Verification items for the finished model (mm, model axes). A direction names the side the tool comes from. Coordinates: 2 decimals unless noted, no trailing zeros. Order: outer loops, then holes, each group sorted by start corner. A loop starts at its lowest first (then second) coordinate and runs counter-clockwise, first axis right, second up. Notation, with made-up numbers: (76.5, 46) -> (107.5, 46) arc R26 ccw to (107.5, 67) -> close; hole circle Ø3 at (79, -7.75). An arc over 180 degrees is marked (long way). Answer as CSV lines item,"result".
```python
from build123d import *

# Parameters (mm, degrees)
SKETCH_W        = 117
SKETCH_H        = 62
SKETCH_R        = 2
SKETCH_R_2      = 12
PAD_DEPTH       = 2
SKETCH001_W     = 114.9
SKETCH001_H     = 57.8
SKETCH001_W_2   = 110.9
SKETCH001_H_2   = 53.8
SKETCH001_W_3   = 2
SKETCH001_H_3   = 2.1
PAD001_DEPTH    = 2
SKETCH003_R     = 2
POCKET_DEPTH    = 2
SKETCH005_W     = 2
SKETCH005_H     = 62
PAD002_DEPTH    = 19.9
SKETCH006_W     = 2
SKETCH006_H     = 17
POCKET001_DEPTH = 15
SKETCH007_W     = 2
SKETCH007_H     = 15
POCKET002_DEPTH = 17
SKETCH008_R     = 4
SKETCH008_R_2   = 2
PAD003_DEPTH    = 2
SKETCH009_R     = 1.5
POCKET003_DEPTH = 5


with BuildPart() as part:
    # Sketch → Pad (new body)
    with BuildSketch(Plane.XY):
        with Locations((58.5, 31)):
            Rectangle(SKETCH_W, SKETCH_H)
        with Locations((38, 43)):
            Circle(SKETCH_R, mode=Mode.SUBTRACT)
        with Locations((62, 43)):
            Circle(SKETCH_R, mode=Mode.SUBTRACT)
        with Locations((38, 19)):
            Circle(SKETCH_R, mode=Mode.SUBTRACT)
        with Locations((62, 19)):
            Circle(SKETCH_R, mode=Mode.SUBTRACT)
        with Locations((50, 31)):
            Circle(SKETCH_R_2, mode=Mode.SUBTRACT)
        with BuildLine():
            ThreePointArc((71.5, 20), (70, 21.5), (68.5, 20))
            Line((68.5, 20), (68.5, 4))
            ThreePointArc((68.5, 4), (70, 2.5), (71.5, 4))
            Line((71.5, 20), (71.5, 4))
        make_face(mode=Mode.SUBTRACT)
    extrude(amount=PAD_DEPTH)

    # Sketch001 (on Face14 of Pad) → Pad001 (join)
    with BuildSketch(Plane(origin=(0, 0, 0), x_dir=(1, 0, 0), z_dir=(0, 0, -1))):
        with Locations((59.55, -31)):
            Rectangle(SKETCH001_W, SKETCH001_H)
        with Locations((59.55, -31)):
            Rectangle(SKETCH001_W_2, SKETCH001_H_2, mode=Mode.SUBTRACT)
        with Locations((116, -1.05)):
            Rectangle(SKETCH001_W_3, SKETCH001_H_3)
        with Locations((116, -60.95)):
            Rectangle(SKETCH001_W_3, SKETCH001_H_3)
    extrude(amount=PAD001_DEPTH)

    # Sketch003 → Pocket (cut)
    with BuildSketch(Plane.XY.offset(2)):
        with Locations((6, 64)):
            Circle(SKETCH003_R)
        with Locations((113, 64)):
            Circle(SKETCH003_R)
        with Locations((6, -2)):
            Circle(SKETCH003_R)
        with Locations((113, -2)):
            Circle(SKETCH003_R)
    extrude(amount=-POCKET_DEPTH, mode=Mode.SUBTRACT)

    # Sketch005 (on Face16 of Pad001) → Pad002 (join)
    with BuildSketch(Plane(origin=(0, 0, -2), x_dir=(1, 0, 0), z_dir=(0, 0, -1))):
        with Locations((116, -31)):
            Rectangle(SKETCH005_W, SKETCH005_H)
    extrude(amount=PAD002_DEPTH)

    # Sketch006 (on Face37 of Pad002) → Pocket001 (cut)
    with BuildSketch(Plane(origin=(0, 0, -21.9), x_dir=(1, 0, 0), z_dir=(0, 0, -1))):
        with Locations((116, -12.5)):
            Rectangle(SKETCH006_W, SKETCH006_H)
    extrude(amount=-POCKET001_DEPTH, mode=Mode.SUBTRACT)

    # Sketch007 (on Face41 of Pocket001) → Pocket002 (cut)
    with BuildSketch(Plane(origin=(0, 0, -21.9), x_dir=(1, 0, 0), z_dir=(0, 0, -1))):
        with Locations((116, -32)):
            Rectangle(SKETCH007_W, SKETCH007_H)
        with Locations((116, -50)):
            Rectangle(SKETCH007_W, SKETCH007_H)
    extrude(amount=-POCKET002_DEPTH, mode=Mode.SUBTRACT)

    # Sketch008 (on Face4 of Pocket002) → Pad003 (join)
    with BuildSketch(Plane.XY.offset(2)):
        with Locations((6, 64)):
            Circle(SKETCH008_R)
        with Locations((6, 64)):
            Circle(SKETCH008_R_2, mode=Mode.SUBTRACT)
        with Locations((111, 64)):
            Circle(SKETCH008_R)
        with Locations((111, 64)):
            Circle(SKETCH008_R_2, mode=Mode.SUBTRACT)
        with Locations((6, -2)):
            Circle(SKETCH008_R)
        with Locations((6, -2)):
            Circle(SKETCH008_R_2, mode=Mode.SUBTRACT)
        with Locations((111, -2)):
            Circle(SKETCH008_R)
        with Locations((111, -2)):
            Circle(SKETCH008_R_2, mode=Mode.SUBTRACT)
    extrude(amount=-PAD003_DEPTH)

    # Sketch009 (on Face59 of Pad003) → Pocket003 (cut)
    with BuildSketch(Plane.XY):
        with Locations((70, 4)):
            Circle(SKETCH009_R)
    extrude(amount=-POCKET003_DEPTH, mode=Mode.SUBTRACT)


solid = part.part
```
Item 1: Section check B-B, the plane x = 70. Record the boundary of the cut face in (y, z), plus the area to 3 significant figures.
Answer list:
outline,"(0, 0) -> (2.1, 0) -> (2.1, -2) -> (2.5, -2) -> (2.5, 2) -> (0, 2) -> close; (21.5, 0) -> (57.9, 0) -> (57.9, -2) -> (59.9, -2) -> (59.9, 0) -> (62, 0) -> (62, 2) -> (21.5, 2) -> close"
area,"90.8 mm2"
Item 2: Section check C-C, the plane z = -14.5. Record the boundary of the cut face in (x, y).
Answer list:
outline,"(115, 0) -> (117, 0) -> (117, 4) -> (115, 4) -> close; (115, 21) -> (117, 21) -> (117, 24.5) -> (115, 24.5) -> close; (115, 39.5) -> (117, 39.5) -> (117, 42.5) -> (115, 42.5) -> close; (115, 57.5) -> (117, 57.5) -> (117, 62) -> (115, 62) -> close"
Item 3: Thickness scan on line 1 (Y direction, x = 6, z = 1.2); line 2 (Z direction, x = 84.5, y = 4); line 3 (Z direction, x = 89, y = 5.5). Record the ranges inside material, lowest first.
Answer list:
line 1,"-6 to -4, 0 to 62, 66 to 68"
line 2,"-2 to 2"
line 3,"0 to 2"
Item 4: Section check D-D, the plane x = 6. Record the boundary of the cut face in (y, z).
Answer list:
outline,"(-6, 0) -> (-4, 0) -> (-4, 2) -> (-6, 2) -> close; (0, 0) -> (2.1, 0) -> (2.1, -2) -> (4.1, -2) -> (4.1, 0) -> (57.9, 0) -> (57.9, -2) -> (59.9, -2) -> (59.9, 0) -> (62, 0) -> (62, 2) -> (0, 2) -> close; (66, 0) -> (68, 0) -> (68, 2) -> (66, 2) -> close"
Item 5: Release check for a two-part mould opening along X. For faces 4 (the flat face through (42, 59, -2)), 5 (the cylindrical face through (62, 41, 1)), 6 (the flat face through (117, 31, -4)) record: +X half, -X half, draft (parallel to the pull), parting line (faces both ways), or undercut.
Answer list:
face 4,"draft"
face 5,"undercut"
face 6,"+X half"
Item 6: Tool access check on faces 1 (the flat face through (71, 32, 2)), 2 (the flat face through (115, 31, -3)), 3 (the cylindrical face through (70, 2.5, 0)). Record the directions out of +Z, -Z, +X, -X, +Y, -Y that give a thin tool (end or side, any length) a straight path to the whole face; none if there is none.
Answer list:
face 1,"+Z, +X, -X, +Y, -Y"
face 2,"-Z"
face 3,"+Z, -Z"
Item 7: Depth check by flat-ended pin: pin 1 Ø3 at (x, y) = (20.5, 34.5) entering from -Z; pin 2 Ø0.6 at (x, z) = (115.5, -12.5) entering from -Y; pin 3 Ø0.6 at (x, z) = (115.5, -14.5) entering from +Y; pin 4 Ø3.5 at (x, y) = (38, 19) entering from -Z. Enter the tip coordinate at first touch or a pass-through.
Answer list:
pin 1,"z = 0"
pin 2,"y = 0"
pin 3,"y = 62"
pin 4,"through"
Item 8: Section check A-A, the plane y = 31. Record the boundary of the cut face in (x, z).
Answer list:
outline,"(0, 0) -> (2.1, 0) -> (2.1, -2) -> (4.1, -2) -> (4.1, 0) -> (38, 0) -> (38, 2) -> (0, 2) -> close; (62, 0) -> (115, 0) -> (115, -4.9) -> (117, -4.9) -> (117, 2) -> (62, 2) -> close"
